The model under review builds one solid part; all positions refer to its coordinate system, in mm. A direction names the side the tool comes from. Round coordinates to 2 decimals unless told otherwise and drop trailing zeros. Write each loop counter-clockwise with the first axis right and the second up, starting at its lowest first coordinate (ties: lowest second). Pieces come first, ordered by that corner, then holes. Notation, with made-up numbers: M 29,-5.75 L 66,-5.75 A17 cw 66,11.25 Z; hole C 43.25,27.5 d5. An arc over 180 degrees is marked long. One line per item, written item: value. Start each with the question number.
1) Wall thickness on probe 1 along X at (y, z) = (-1.15, 3.5); probe 2 along Y at (x, z) = (3.5, 9.25): over which ranges is each line inside the solid? List them lowest first.
2) Take a section at A-A, the plane z = 3.5. Write out the cut boundary in (x, y), and give its area (3 significant figures).
3) For P1, Ø1.6, axis at x = 30, y = 10, coming from the -Z side; P2, Ø1.6, axis at x = 18, y = 29.5, coming from the +Z side, all flat-tipped, find the tip position at first contact; note any pin that passes through.
4) Take a section at B-B, the plane y = 1. Write out the cut boundary in (x, z), and give its area (3 significant figures).
5) Take a section at C-C, the plane x = 9.5. Write out the cut boundary in (y, z).
6) Tool access review of faces 1 (the face through (14, 30, 0)), 2 (the face through (29, 14, 9)), 3 (the face through (7, 30, 12)), 4 (the face through (10.44, -1.01, 2.27)), 5 (the face through (30, 9, 5)): name each direction out of +Z, -Z, +X, -X, +Y, -Y from which nothing blocks a thin tool from reaching the whole face with its end or side.
7) Mouldability with a two-part tool opening along Y and no side actions: class faces 6 (the face through (14, 29, 6)), 7 (the face through (22, 30, 12)), 8 (the face through (14, 31, 6)), 9 (the face through (-1, 9, 5)) as +Y half, -Y half, draft (parallel to the pull), parting line (faces both ways), or undercut.
from build123d import *

# Parameters (mm, degrees)
SKETCH_1_W               = 33
SKETCH_1_H               = 33
SKETCH_1_W_2             = 29
SKETCH_1_H_2             = 29
EXTRUDE_1_DEPTH          = 14.5
CUT_EXTRUDE_2_REACH      = 49.542
SKETCH_3_W               = 15
SKETCH_3_H               = 6
CUT_EXTRUDE_4_REACH      = 49.542
SKETCH_5_R               = 1.55
CUT_EXTRUDE_5_DEPTH      = 48.542086618
CUT_EXTRUDE_5_DEPTH_BACK = 48.542086618
SKETCH_6_W               = 5
SKETCH_6_H               = 10


with BuildPart() as part:
    # 草图1 → 凸台-拉伸1 (new body)
    with BuildSketch(Plane.XY):
        with Locations((14.5, 14.5)):
            Rectangle(SKETCH_1_W, SKETCH_1_H)
        with Locations((14.5, 14.5)):
            Rectangle(SKETCH_1_W_2, SKETCH_1_H_2, mode=Mode.SUBTRACT)
    extrude(amount=EXTRUDE_1_DEPTH)

    # 草图3 → 切除-拉伸2 (cut, up to next)
    with BuildSketch(Plane(origin=(0, 31, 0), x_dir=(1, 0, 0), z_dir=(0, 1, 0)), mode=Mode.PRIVATE) as cut_extrude_2_sk1:
        with Locations((14.5, -11.5)):
            Rectangle(SKETCH_3_W, SKETCH_3_H)
    cut_extrude_2_tool1 = extrude(cut_extrude_2_sk1.sketch, amount=-CUT_EXTRUDE_2_REACH, mode=Mode.PRIVATE) & part.part
    add(cut_extrude_2_tool1.solids().sort_by_distance((14.5, 31, 11.5))[0], mode=Mode.SUBTRACT)

    # 草图5 → 切除-拉伸4 (cut, up to next)
    with BuildSketch(Plane.XZ.offset(2), mode=Mode.PRIVATE) as cut_extrude_4_sk1:
        with Locations(Location((19.5, 3.5, 0), (0, 0, 270))):
            Circle(SKETCH_5_R)
    cut_extrude_4_tool1 = extrude(cut_extrude_4_sk1.sketch, amount=-CUT_EXTRUDE_4_REACH, mode=Mode.PRIVATE) & part.part
    # 草图5 → 切除-拉伸4 (cut, up to next)
    with BuildSketch(Plane.XZ.offset(2), mode=Mode.PRIVATE) as cut_extrude_4_sk2:
        with Locations(Location((9.5, 3.5, 0), (0, 0, 90))):
            Circle(SKETCH_5_R)
    cut_extrude_4_tool2 = extrude(cut_extrude_4_sk2.sketch, amount=-CUT_EXTRUDE_4_REACH, mode=Mode.PRIVATE) & part.part
    add(cut_extrude_4_tool1.solids().sort_by_distance((19.5, -2, 3.5))[0], mode=Mode.SUBTRACT)
    add(cut_extrude_4_tool2.solids().sort_by_distance((9.5, -2, 3.5))[0], mode=Mode.SUBTRACT)

    # 草图6 → 切除-拉伸5 (cut, two sides: drawn at the far end of the back side and taken through both)
    with BuildSketch(Plane.ZY.offset(2).offset(-CUT_EXTRUDE_5_DEPTH_BACK)):
        with Locations((2.5, 9.5)):
            Rectangle(SKETCH_6_W, SKETCH_6_H)
    extrude(amount=CUT_EXTRUDE_5_DEPTH + CUT_EXTRUDE_5_DEPTH_BACK, mode=Mode.SUBTRACT)


solid = part.part
Checked values:
1. probe 1: x = -2 to 7.95, 11.05 to 17.95, 21.05 to 31
1. probe 2: y = -2 to 0, 29 to 31
2. outline: M -2,-2 L 7.95,-2 L 7.95,0 L 0,0 L 0,4.5 L -2,4.5 Z; M -2,14.5 L 0,14.5 L 0,29 L 29,29 L 29,14.5 L 31,14.5 L 31,31 L -2,31 Z; M 11.05,-2 L 17.95,-2 L 17.95,0 L 11.05,0 Z; M 21.05,-2 L 31,-2 L 31,4.5 L 29,4.5 L 29,0 L 21.05,0 Z
2. area: 196 mm2
3. P1: stops at z = 5
3. P2: stops at z = 8.5
4. outline: M -2,0 L 0,0 L 0,14.5 L -2,14.5 Z; M 29,0 L 31,0 L 31,14.5 L 29,14.5 Z
4. area: 58.0 mm2
5. outline: M -2,0 L 0,0 L 0,1.95 L -2,1.95 Z; M -2,5.05 L 0,5.05 L 0,14.5 L -2,14.5 Z; M 29,0 L 31,0 L 31,8.5 L 29,8.5 Z
6. face 1: -Z, +X, -X, +Y, -Y
6. face 2: +Z, -Z
6. face 3: +Z, +Y
6. face 4: -Y
6. face 5: -Z, +X, -X
7. face 6: undercut
7. face 7: draft
7. face 8: +Y half
7. face 9: undercut
